Here's how the part is built. I have some questions about the finished solid (model axes, mm). A direction names the side the tool comes from. Give positions to 0.01 mm unless a question says otherwise; leave off trailing zeros. Write each loop counter-clockwise with the first axis right and the second up, starting at its lowest first coordinate (ties: lowest second). Pieces come first, ordered by that corner, then holes. Notation, with made-up numbers: (2.5, 84.25) -> (6.5, 84.25) arc R14 ccw to (6.5, 111.25) -> close; hole circle Ø3 at (-35.75, -22). An arc over 180 degrees is marked (long way). Use one line per item in the form item = value.
```python
from build123d import *

# Parameters (mm, degrees)
F0_W          = 150
F0_H          = 40
F1_DEPTH      = 50
F2_T          = -2.5
F5_R          = 2.5
F7_DEPTH      = 40
F6_R          = 2.5
F8_DEPTH      = 40
F4_R          = 2.5
F9_DEPTH      = 40
F3_R          = 2.5
F10_DEPTH     = 40
F11_W         = 150
F11_H         = 50
F12_DEPTH     = 10
F13_W         = 45
F13_H         = 20
F14_DEPTH     = 25
F15_W         = 44.8060352355
F15_H         = 19.2025862634
F16_DEPTH     = 10
F17_W         = 25
F17_H         = 8
F18_DEPTH     = 25
F19_R         = 15
F20_DEPTH     = 5
F21_R         = 5
F22_T1_DEPTH  = 57.5
F22_T3_DEPTH  = 40
F22_T5_DEPTH  = 57.5
F22_T7_DEPTH  = 40
F22_S11_W     = 5
F22_S11_H     = 5
F22_T12_DEPTH = 5
F22_S17_W     = 5
F22_S17_H     = 5
F22_T18_DEPTH = 5
F22_S23_W     = 5
F22_S23_H     = 5
F22_T24_DEPTH = 5
F22_S29_W     = 5
F22_S29_H     = 5
F22_T30_DEPTH = 5
F22_T34_ANGLE = 90
F22_T36_ANGLE = 90
F22_T38_ANGLE = 90
F23_T1_DEPTH  = 62.5
F23_S5_W      = 5
F23_S5_H      = 5
F23_T6_DEPTH  = 5
F24_W         = 60
F24_H         = 10
F25_DEPTH     = 25


# Not quite as in the source:
# - a fillet or chamfer that OpenCascade refuses, or shapes differently, is made with other operations: its cross-section is extruded or revolved along the edge and cut away or added


with BuildPart() as f1:
    # F0 (on Front) → F1 (new body)
    with BuildSketch(Plane.XZ):
        with Locations((-1.4870658517, -2.6939674467)):
            Rectangle(F0_W, F0_H)
    extrude(amount=F1_DEPTH)

    # F2
    f2_openings = [f1.faces().sort_by_distance(p)[0] for p in [
        (-1.487066, -25, 17.306033),
    ]]
    offset(amount=F2_T, openings=f2_openings)

    # F5 (on face) → F7 (join)
    with BuildSketch(Plane.XY.offset(-20.1939674467)):
        with Locations((64.5129341483, -42)):
            Circle(F5_R)
    extrude(amount=F7_DEPTH)

    # F6 (on face) → F8 (join)
    with BuildSketch(Plane.XY.offset(-20.1939674467)):
        with Locations((-67.4870658517, -42)):
            Circle(F6_R)
    extrude(amount=F8_DEPTH)

    # F4 (on face) → F9 (join)
    with BuildSketch(Plane.XY.offset(-20.1939674467)):
        with Locations((64.5129341483, -8)):
            Circle(F4_R)
    extrude(amount=F9_DEPTH)

    # F3 (on face) → F10 (join)
    with BuildSketch(Plane.XY.offset(-20.1939674467)):
        with Locations((-67.4870658517, -8)):
            Circle(F3_R)
    extrude(amount=F10_DEPTH)

    # F11 (on face) → F12 (join)
    with BuildSketch(Plane.XY.offset(17.3060325533)):
        with Locations((-1.4870658517, -25)):
            Rectangle(F11_W, F11_H)
    extrude(amount=F12_DEPTH)

    # F13 (on face) → F14 (cut)
    with BuildSketch(Plane.XY.offset(27.3060325533)):
        with Locations((-3.9870658517, -40)):
            Rectangle(F13_W, F13_H)
    extrude(amount=-F14_DEPTH, mode=Mode.SUBTRACT)

    # F15 (on Top) → F16 (join)
    with BuildSketch(Plane.XY):
        with Locations((-4.1379285976, -39.8599151522)):
            Rectangle(F15_W, F15_H)
    extrude(amount=F16_DEPTH)

    # F17 (on face) → F18 (cut)
    with BuildSketch(Plane.XY.offset(10)):
        with Locations((-4.5150823891, -41.0000055134)):
            Rectangle(F17_W, F17_H)
    extrude(amount=-F18_DEPTH, mode=Mode.SUBTRACT)

    # F19 (on face) → F20 (cut)
    with BuildSketch(Plane.XZ.offset(50)):
        with Locations((-49.0409471095, 2.3060325533)):
            Circle(F19_R)
        with Locations((43.5129341483, 2.3060325533)):
            Circle(F19_R)
    extrude(amount=-F20_DEPTH, mode=Mode.SUBTRACT)

    # F21
    f21_edges = [f1.edges().sort_by_distance(p)[0] for p in [
        (-1.487066, -50, -22.693967),
        (73.512934, -25, -22.693967),
        (-76.487066, -25, -22.693967),
        (-1.487066, 0, -22.693967),
        (-1.487066, 0, 27.306033),
        (-51.487066, -50, 27.306033),
    ]]
    fillet(f21_edges, radius=F21_R)

    # F22: fillet of radius 5 on 3 edges, made by hand

    # F22_s2 → F22_t1 (cut)
    with BuildSketch(Plane.XZ.offset(5)):
        with BuildLine():
            ThreePointArc((68.5129341483, 27.3060325533), (72.0484680542, 25.8415664592), (73.5129341483, 22.3060325533))
            Line((73.5129341483, 22.3060325533), (73.5129341483, 27.3060325533))
            Line((73.5129341483, 27.3060325533), (68.5129341483, 27.3060325533))
        make_face()
    extrude(amount=F22_T1_DEPTH, mode=Mode.SUBTRACT)

    # F22_s4 → F22_t3 (cut)
    with BuildSketch(Plane.XZ.offset(5)):
        with BuildLine():
            ThreePointArc((-76.4870658517, 22.3060325533), (-75.0225997576, 25.8415664592), (-71.4870658517, 27.3060325533))
            Line((-71.4870658517, 27.3060325533), (-76.4870658517, 27.3060325533))
            Line((-76.4870658517, 27.3060325533), (-76.4870658517, 22.3060325533))
        make_face()
    extrude(amount=F22_T3_DEPTH, mode=Mode.SUBTRACT)

    # F22_s6 → F22_t5 (cut)
    with BuildSketch(Plane.XY.offset(-17.6939674467)):
        with BuildLine():
            ThreePointArc((68.5129341483, -50), (72.0484680542, -48.5355339059), (73.5129341483, -45))
            Line((73.5129341483, -45), (73.5129341483, -50))
            Line((73.5129341483, -50), (68.5129341483, -50))
        make_face()
    extrude(amount=F22_T5_DEPTH, mode=Mode.SUBTRACT)

    # F22_s8 → F22_t7 (cut)
    with BuildSketch(Plane.XY.offset(-17.6939674467)):
        with BuildLine():
            ThreePointArc((-76.4870658517, -45), (-75.0225997576, -48.5355339059), (-71.4870658517, -50))
            Line((-71.4870658517, -50), (-76.4870658517, -50))
            Line((-76.4870658517, -50), (-76.4870658517, -45))
        make_face()
        with BuildLine():
            ThreePointArc((-76.4870658517, -5), (-75.0225997576, -1.4644660941), (-71.4870658517, 0))
            Line((-71.4870658517, 0), (-76.4870658517, 0))
            Line((-76.4870658517, 0), (-76.4870658517, -5))
        make_face()
        with BuildLine():
            ThreePointArc((68.5129341483, 0), (72.0484680542, -1.4644660941), (73.5129341483, -5))
            Line((73.5129341483, -5), (73.5129341483, 0))
            Line((73.5129341483, 0), (68.5129341483, 0))
        make_face()
    extrude(amount=F22_T7_DEPTH, mode=Mode.SUBTRACT)


with BuildPart() as f22_tool10:
    # F22_s11 → F22_t12 (new body)
    with BuildSketch(Plane.XZ.offset(45)):
        with Locations((71.0129341483, -20.1939674467)):
            Rectangle(F22_S11_W, F22_S11_H)
    extrude(amount=F22_T12_DEPTH)

    # F22_s13 → F22_t14 (revolve, cut)
    with BuildSketch(Plane(origin=(68.5129341483, -45, -17.6939674467), x_dir=(-0.7071067812, 0, 0.7071067812), z_dir=(0.7071067812, 0, 0.7071067812))):
        with BuildLine():
            ThreePointArc((0, -5), (5, 0), (0, 5))
            Line((0, 5), (0, -5))
        make_face()
    revolve(axis=Axis((68.5129341483, -45, -17.6939674467), (0, -1, 0)), mode=Mode.SUBTRACT)


with BuildPart() as f1_1:
    add(f1.part)

    # F22_t9: cut F22_tool10
    add(f22_tool10.part, mode=Mode.SUBTRACT)


with BuildPart() as f22_tool16:
    # F22_s17 → F22_t18 (new body)
    with BuildSketch(Plane.YZ.offset(-71.4870658517)):
        with Locations((-47.5, -20.1939674467)):
            Rectangle(F22_S17_W, F22_S17_H)
    extrude(amount=-F22_T18_DEPTH)

    # F22_s19 → F22_t20 (revolve, cut)
    with BuildSketch(Plane(origin=(-71.4870658517, -45, -17.6939674467), x_dir=(0, 0.7071067812, 0.7071067812), z_dir=(0, -0.7071067812, 0.7071067812))):
        with BuildLine():
            ThreePointArc((0, -5), (5, 0), (0, 5))
            Line((0, 5), (0, -5))
        make_face()
    revolve(axis=Axis((-71.4870658517, -45, -17.6939674467), (-1, 0, 0)), mode=Mode.SUBTRACT)


with BuildPart() as f1_2:
    add(f1_1.part)

    # F22_t15: cut F22_tool16
    add(f22_tool16.part, mode=Mode.SUBTRACT)


with BuildPart() as f22_tool22:
    # F22_s23 → F22_t24 (new body)
    with BuildSketch(Plane.YZ.offset(-71.4870658517)):
        with Locations((-2.5, -20.1939674467)):
            Rectangle(F22_S23_W, F22_S23_H)
    extrude(amount=-F22_T24_DEPTH)

    # F22_s25 → F22_t26 (revolve, cut)
    with BuildSketch(Plane(origin=(-71.4870658517, -5, -17.6939674467), x_dir=(0, -0.7071067812, 0.7071067812), z_dir=(0, -0.7071067812, -0.7071067812))):
        with BuildLine():
            ThreePointArc((0, -5), (5, 0), (0, 5))
            Line((0, 5), (0, -5))
        make_face()
    revolve(axis=Axis((-71.4870658517, -5, -17.6939674467), (-1, 0, 0)), mode=Mode.SUBTRACT)


with BuildPart() as f1_3:
    add(f1_2.part)

    # F22_t21: cut F22_tool22
    add(f22_tool22.part, mode=Mode.SUBTRACT)


with BuildPart() as f22_tool28:
    # F22_s29 → F22_t30 (new body)
    with BuildSketch(Plane.XZ.offset(5)):
        with Locations((71.0129341483, -20.1939674467)):
            Rectangle(F22_S29_W, F22_S29_H)
    extrude(amount=-F22_T30_DEPTH)

    # F22_s31 → F22_t32 (revolve, cut)
    with BuildSketch(Plane(origin=(68.5129341483, -5, -17.6939674467), x_dir=(-0.7071067812, 0, 0.7071067812), z_dir=(-0.7071067812, 0, -0.7071067812))):
        with BuildLine():
            ThreePointArc((0, -5), (5, 0), (0, 5))
            Line((0, 5), (0, -5))
        make_face()
    revolve(axis=Axis((68.5129341483, -5, -17.6939674467), (0, 1, 0)), mode=Mode.SUBTRACT)


with BuildPart() as f1_4:
    add(f1_3.part)

    # F22_t27: cut F22_tool28
    add(f22_tool28.part, mode=Mode.SUBTRACT)

    # F22_s33 → F22_t34 (revolve, cut)
    with BuildSketch(Plane.XY.offset(22.3060325533)):
        with BuildLine():
            ThreePointArc((-76.4870658517, -5), (-75.0225997576, -1.4644660941), (-71.4870658517, 0))
            Line((-71.4870658517, 0), (-76.4870658517, 0))
            Line((-76.4870658517, 0), (-76.4870658517, -5))
        make_face()
    revolve(axis=Axis((-76.4870658517, -5, 22.3060325533), (1, 0, 0)), revolution_arc=F22_T34_ANGLE, mode=Mode.SUBTRACT)

    # F22_s35 → F22_t36 (revolve, cut)
    with BuildSketch(Plane.XZ.offset(45)):
        with BuildLine():
            ThreePointArc((-76.4870658517, 22.3060325533), (-75.0225997576, 25.8415664592), (-71.4870658517, 27.3060325533))
            Line((-71.4870658517, 27.3060325533), (-76.4870658517, 27.3060325533))
            Line((-76.4870658517, 27.3060325533), (-76.4870658517, 22.3060325533))
        make_face()
    revolve(axis=Axis((-76.4870658517, -45, 22.3060325533), (1, 0, 0)), revolution_arc=F22_T36_ANGLE, mode=Mode.SUBTRACT)

    # F22_s37 → F22_t38 (revolve, cut)
    with BuildSketch(Plane.XY.offset(22.3060325533)):
        with BuildLine():
            ThreePointArc((68.5129341483, 0), (72.0484680542, -1.4644660941), (73.5129341483, -5))
            Line((73.5129341483, -5), (73.5129341483, 0))
            Line((73.5129341483, 0), (68.5129341483, 0))
        make_face()
    revolve(axis=Axis((73.5129341483, -5, 22.3060325533), (1, 0, 0)), revolution_arc=F22_T38_ANGLE, mode=Mode.SUBTRACT)

    # F23: fillet of radius 5 on 1 edges, made by hand

    # F23_s2 → F23_t1 (cut)
    with BuildSketch(Plane.YZ.offset(6.0129341483)):
        with BuildLine():
            ThreePointArc((-50, 22.3060325533), (-48.5355339059, 25.8415664592), (-45, 27.3060325533))
            Line((-45, 27.3060325533), (-50, 27.3060325533))
            Line((-50, 27.3060325533), (-50, 22.3060325533))
        make_face()
    extrude(amount=F23_T1_DEPTH, mode=Mode.SUBTRACT)


with BuildPart() as f23_tool4:
    # F23_s5 → F23_t6 (new body)
    with BuildSketch(Plane.XZ.offset(45)):
        with Locations((71.0129341483, 24.8060325533)):
            Rectangle(F23_S5_W, F23_S5_H)
    extrude(amount=F23_T6_DEPTH)

    # F23_s7 → F23_t8 (revolve, cut)
    with BuildSketch(Plane(origin=(68.5129341483, -45, 22.3060325533), x_dir=(-0.7071067812, 0, -0.7071067812), z_dir=(-0.7071067812, 0, 0.7071067812))):
        with BuildLine():
            ThreePointArc((0, -5), (5, 0), (0, 5))
            Line((0, 5), (0, -5))
        make_face()
    revolve(axis=Axis((68.5129341483, -45, 22.3060325533), (0, -1, 0)), mode=Mode.SUBTRACT)


with BuildPart() as f1_5:
    add(f1_4.part)

    # F23_t3: cut F23_tool4
    add(f23_tool4.part, mode=Mode.SUBTRACT)

    # F24 (on face) → F25 (cut)
    with BuildSketch(Plane.XZ.offset(50)):
        with Locations((-2.7640064806, -7.5991895379)):
            Rectangle(F24_W, F24_H)
    extrude(amount=-F25_DEPTH, mode=Mode.SUBTRACT)


solid = f1_5.part
```
Q1. Will these pins go through, and if not, where does the flat tip stop? pin 1 Ø15.5 at (x, y) = (0, -39.5) entering from +Z; pin 2 Ø0.8 at (y, z) = (-48, -6.5) entering from +X; pin 3 Ø2 at (x, y) = (1.5, -49.5) entering from -Z.
Result set:
pin_1 = 10
pin_2 = 72.78
pin_3 = -21.26
Q2. Which directions (+Z, -Z, +X, -X, +Y, -Y) give clear straight access to the entire face, cutting with the end or side of a thin tool? Please do faces 1 (the face through (-3, -47.5, -1)), 2 (the face through (27.236, -49, -8)), 3 (the face through (-4, -49.461, 6)), 4 (the face through (-5, -37, 5)).
Result set:
face_1 = none
face_2 = -Y
face_3 = +Z, -Y
face_4 = +Z
Q3. I want a section at D-D, the plane y = -33. Write out the boundary of the cut face in (x, z).
Result set:
outline = (-76.49, -17.69) arc R5 ccw to (-71.49, -22.69) -> (68.51, -22.69) arc R5 ccw to (73.51, -17.69) -> (73.51, 22.31) arc R5 ccw to (68.51, 27.31) -> (18.51, 27.31) -> (18.51, 17.31) -> (71.01, 17.31) -> (71.01, -20.19) -> (-73.99, -20.19) -> (-73.99, 17.31) -> (-26.49, 17.31) -> (-26.49, 27.31) -> (-71.49, 27.31) arc R5 ccw to (-76.49, 22.31) -> close; (-26.54, 0) -> (18.27, 0) -> (18.27, 10) -> (-26.54, 10) -> close
Q4. If I drill on line 1 along Y through (x, z) = (-16, 0.5); line 2 along Y through (x, z) = (2.5, 8); line 3 along X through (y, z) = (-45.5, 4.5), over which ranges is the centre line in solid material (lowest first)? Write a range as from..to.
Result set:
line_1 = -50..-45, -37..-30.26, -2.5..0
line_2 = -49.46..-45, -37..-30.26, -2.5..0
line_3 = -76.46..-73.99, -26.54..18.27, 71.01..73.49
Q5. If we mould it in two halves opening along X, with no side actions, what happens to faces 5 (the face through (-75.06, -25.28, -21.19)), 6 (the face through (-2, -25, 27.306)), 7 (the face through (-26.541, -39, 5))? For each: +X half, -X half, draft (parallel to the pull), parting line (faces both ways), or undercut.
Result set:
face_5 = -X half
face_6 = draft
face_7 = undercut
Q6. I want a section at A-A, the plane y = -42. Count the separate pieces of the cut face and the enclosed holes in it, and give its area (3 significant figures).
Result set:
separate_pieces = 3
enclosed_holes = 2
area = 2,160 mm2
Q7. I want a section at B-B, the plane x = -7.5. Write out the boundary of the cut face in (y, z).
Result set:
outline = (-50, -17.69) arc R5 ccw to (-45, -22.69) -> (-5, -22.69) arc R5 ccw to (0, -17.69) -> (0, 22.31) arc R5 ccw to (-5, 27.31) -> (-30, 27.31) -> (-30, 17.31) -> (-2.5, 17.31) -> (-2.5, -20.19) -> (-47.5, -20.19) -> (-47.5, -12.6) -> (-50, -12.6) -> close; (-50, -2.6) -> (-47.5, -2.6) -> (-47.5, 0) -> (-45, 0) -> (-45, 10) -> (-49.46, 10) -> (-49.46, 2.31) -> (-50, 2.31) -> close; (-37, 0) -> (-30.26, 0) -> (-30.26, 10) -> (-37, 10) -> close
Q8. I want a section at C-C, the plane z = 11.5. Write out the boundary of the cut face in (x, y), and give its area (3 significant figures).
Result set:
outline = (-76.49, -45) arc R5 ccw to (-71.49, -50) -> (-60.89, -50) -> (-60.89, -47.5) -> (-73.99, -47.5) -> (-73.99, -2.5) -> (71.01, -2.5) -> (71.01, -47.5) -> (55.36, -47.5) -> (55.36, -50) -> (68.51, -50) arc R5 ccw to (73.51, -45) -> (73.51, -5) arc R5 ccw to (68.51, 0) -> (-71.49, 0) arc R5 ccw to (-76.49, -5) -> close; circle Ø5 at (-67.49, -42); circle Ø5 at (-67.49, -8); (-37.19, -50) -> (-26.49, -50) -> (-26.49, -47.5) -> (-37.19, -47.5) -> close; (18.51, -50) -> (31.66, -50) -> (31.66, -47.5) -> (18.51, -47.5) -> close; circle Ø5 at (64.51, -42); circle Ø5 at (64.51, -8)
area = 801 mm2
